Source: CAD feature listing. Evaluate the final solid. Frame: model axes, mm. Face numbers are marked on the shaded views. Coordinates: 2 decimals unless noted, no trailing zeros. Write each loop counter-clockwise with the first axis right and the second up, starting at its lowest first coordinate (ties: lowest second). Pieces come first, ordered by that corner, then holes. Notation, with made-up numbers: (-10.5, -27) -> (11.5, -27) arc R13 cw to (11.5, -10) -> close; hole circle Ø11 at (-29, -21.75). An arc over 180 degrees is marked (long way). Write item = value, one per line.
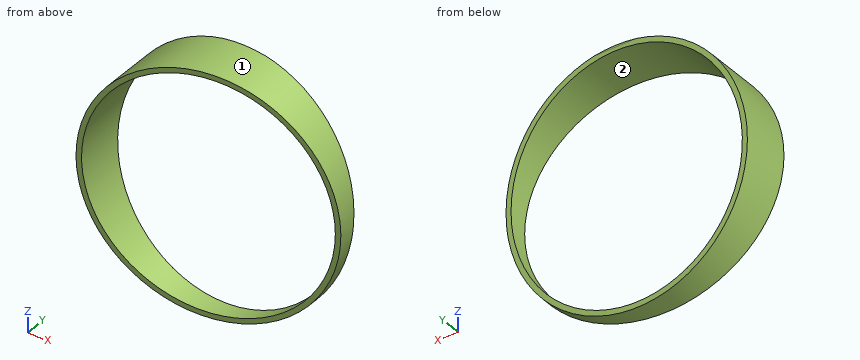
from build123d import *

# Parameters (mm, degrees)
F0_R     = 38.1
F0_R_2   = 36.5125
F1_DEPTH = 12.7
F5_DEPTH = 38.1
F8_DEPTH = 50.8


with BuildPart() as f1:
    # F0 (on Front) → F1 (new body, symmetric)
    with BuildSketch(Plane.XZ):
        with Locations((0, 38.1)):
            Circle(F0_R)
        with Locations((0, 38.1)):
            Circle(F0_R_2, mode=Mode.SUBTRACT)
    extrude(amount=F1_DEPTH, both=True)

    # F4 (on Right) → F5 (cut, symmetric)
    with BuildSketch(Plane.YZ):
        Polygon((12.7786435187, -8.8192215189), (12.7786435187, 76.2), (1.5856506628, -8.8192215189), align=None)
    extrude(amount=F5_DEPTH, both=True, mode=Mode.SUBTRACT)

    # F7 (on offset) → F8 (cut, symmetric)
    with BuildSketch(Plane(origin=(2.1557702546, 0.302973751, 0), x_dir=(0.139173101, -0.9902680687, 0), z_dir=(-0.9902680687, -0.139173101, 0))):
        Polygon((31.6142430529, 76.0232245399), (3.0474591767, 76.5205744021), (3.0474591767, -2.2310584007), (31.6142430529, -2.2310584007), align=None)
    extrude(amount=F8_DEPTH, both=True, mode=Mode.SUBTRACT)


solid = f1.part
1) Cut plane C-C, the plane x = 1. Output: boundary loops of the cut face in (y, z).
Answer block:
outline = (-2.94, 0.01) -> (2.75, 0.01) -> (2.96, 1.6) -> (-2.94, 1.6) -> close; (-2.94, 74.6) -> (12.57, 74.6) -> (12.7, 75.6) -> (12.7, 76.19) -> (-2.94, 76.19) -> close
2) Cut plane A-A, the plane z = 37. Output: boundary loops of the cut face in (x, y), and give its area (3 significant figures).
Answer block:
outline = (-38.08, -8.43) -> (-36.5, -8.21) -> (-36.5, 7.62) -> (-38.08, 7.62) -> close; (36.5, 2.05) -> (38.08, 2.27) -> (38.08, 7.62) -> (36.5, 7.62) -> close
area = 34.0 mm2
3) Cut plane D-D, the plane y = -0.25. Output: boundary loops of the cut face in (x, z) (1 decimal), and give its area (3 significant figures).
Answer block:
outline = (20.1, 5.7) -> (20.1, 7.6) arc R36.5 cw (long way) to (20.1, 68.6) -> (20.1, 70.5) arc R38.1 ccw (long way) to start
area = 254 mm2
4) First-contact query: pin 1 Ø12 at (y, z) = (-4, 26) entering from -X; pin 2 Ø12 at (x, z) = (20, 63) entering from +Y; pin 3 Ø1.5 at (x, y) = (-15, -5) entering from +Z. Flat tips, straight axial feed; report the tip coordinate or a pass-through.
Answer block:
pin_1 = -37.61
pin_2 = 11.83
pin_3 = 73.43
5) Material intervals for probe 1 along Z at (x, y) = (0, -1); probe 2 along X at (y, z) = (2.5, 38.1); probe 3 along X at (y, z) = (-1, 39), sorted ascending. Write a range as [from, to].
Answer block:
probe_1 = [0, 1.59], [74.61, 76.2]
probe_2 = [-38.1, -36.51], [36.51, 38.1]
probe_3 = [-38.09, -36.5]
6) Cut plane B-B, the plane x = -8. Output: boundary loops of the cut face in (y, z), and give its area (3 significant figures).
Answer block:
outline = (-4.2, 0.85) -> (2.86, 0.85) -> (3.07, 2.47) -> (-4.2, 2.47) -> close; (-4.2, 73.73) -> (12.45, 73.73) -> (12.67, 75.35) -> (-4.2, 75.35) -> close
area = 38.9 mm2
7) Pull-direction query (X, two-part tool) for the marked faces 1 and 2; classes: +X half, -X half, draft (parallel to the pull), parting line (faces both ways), or undercut.
Answer block:
face_1 = parting line
face_2 = undercut
